from build123d import *

# Parameters (mm, degrees)
F0_W     = 70
F0_H     = 80
F1_DEPTH = 20
F3_DEPTH = 25
F4_R     = 2.5
F5_DEPTH = 25
F6_W     = 10
F6_H     = 25
F7_DEPTH = 79.4


with BuildPart() as f1:
    # F0 (on Front) → F1 (new body, symmetric)
    with BuildSketch(Plane.XZ):
        Rectangle(F0_W, F0_H)
    extrude(amount=F1_DEPTH, both=True)

    # F2 (on face) → F3 (join)
    with BuildSketch(Plane.XY.offset(40)):
        Polygon((22.5, 0), (10.509629, 10), (-10.509629, 10), (-22.5, 0), (-10.509629, -10), (10.509629, -10), align=None)
    extrude(amount=F3_DEPTH)

    # F4 (on face) → F5 (join)
    with BuildSketch(Plane.XY.offset(65)):
        with Locations((-10.509629, 0)):
            Circle(F4_R)
        with Locations((10.509629, 0)):
            Circle(F4_R)
    extrude(amount=F5_DEPTH)

    # F6 (on Top) → F7 (cut)
    with BuildSketch(Plane.XY):
        with Locations((-20.256918, 0)):
            Rectangle(F6_W, F6_H)
    extrude(amount=-F7_DEPTH, mode=Mode.SUBTRACT)


solid = f1.part
Geometry check sheet. Reference: the model listing, model coordinates, mm. A direction names the side the tool comes from. Give positions to 0.01 mm unless a question says otherwise; leave off trailing zeros. Order: outer loops, then holes, each group sorted by start corner. A loop starts at its lowest first (then second) coordinate and runs counter-clockwise, first axis right, second up.
1) Tool access check on faces 5 (the cylindrical face through (12.894, 0.751, 77.325)), 6 (the flat face through (-16.42, 5.07, 52.32)), 7 (the flat face through (0, -10, 52)), 8 (the flat face through (16.59, 4.93, 52.32)), 9 (the flat face through (16.42, -5.07, 52.32)). Record the directions out of +Z, -Z, +X, -X, +Y, -Y that give a thin tool (end or side, any length) a straight path to the whole face; none if there is none.
Results are:
face 5: +Z
face 6: +Z, -X, +Y
face 7: +Z, +X, -X, -Y
face 8: +Z, +X, +Y
face 9: +Z, +X, -Y
2) Cross-section at D-D (y = -4). Record the boundary of the cut face in (x, z), then the cut area to 3 significant figures.
Results are:
outline: (-35, -40) - (-25.26, -40) - (-25.26, 0) - (-15.26, 0) - (-15.26, -40) - (35, -40) - (35, 40) - (17.7, 40) - (17.7, 65) - (-17.7, 65) - (-17.7, 40) - (-35, 40) - close
area: 6,090 mm2
3) Draft check along Y on faces 1 (the flat face through (35, 0, -1)), 2 (the flat face through (-20, 0, 0)), 3 (the flat face through (0, 10, 52)), 4 (the flat face through (-20, 12.5, -20)). Enter one of: released by +Y, released by -Y, zero draft, split by the parting line, or undercut.
Results are:
face 1: zero draft
face 2: undercut
face 3: released by +Y
face 4: undercut
4) Cross-section at A-A (z = -4). Record the boundary of the cut face in (x, y), then the cut area to 3 significant figures.
Results are:
outline: (-35, -20) - (35, -20) - (35, 20) - (-35, 20) - close; hole (-25.26, -12.5) - (-15.26, -12.5) - (-15.26, 12.5) - (-25.26, 12.5) - close
area: 2,550 mm2
5) Cross-section at B-B (x = 6). Record the boundary of the cut face in (y, z), then the cut area to 3 significant figures.
Results are:
outline: (-20, -40) - (20, -40) - (20, 40) - (10, 40) - (10, 65) - (-10, 65) - (-10, 40) - (-20, 40) - close
area: 3,700 mm2
6) Material ranges on probe 1 along X at (y, z) = (-5, -18.5); probe 2 along Y at (x, z) = (-24.5, -15.5); probe 3 along Z at (x, y) = (30.5, 11.5), recorded low to high.
Results are:
probe 1: x = -35 to -25.26, -15.26 to 35
probe 2: y = -20 to -12.5, 12.5 to 20
probe 3: z = -40 to 40
7) Gauge pin test, flat ends, axial feed: pin 1 (1 mm diameter, centred on x = -25.5, y = 5.5, fed in from +Z); pin 2 (4 mm diameter, centred on y = -5.5, z = 54.5, fed in from +X); pin 3 (22 mm diameter, centred on x = -9, y = 3, fed in from +Z); pin 4 (3 mm diameter, centred on x = -19.5, y = 6, fed in from -Z). Record the tip position at first contact, or that the pin passes through.
Results are:
pin 1: stops at z = 40
pin 2: stops at x = 18.3
pin 3: stops at z = 90
pin 4: stops at z = 0
8) Cross-section at C-C (z = 77.5). Record the boundary of the cut face in (x, y), then the cut area to 3 significant figures.
Results are:
outline: circle Ø5 at (-10.51, 0); circle Ø5 at (10.51, 0)
area: 39.3 mm2
